Answer from the drawing. Dimensions are ordinates in mm from the lowest x, y and z of the part. Round coordinates to 2 decimals unless told otherwise and drop trailing zeros. Write each loop counter-clockwise with the first axis right and the second up, starting at its lowest first coordinate (ties: lowest second). Pieces come first, ordered by that corner, then holes.
1. Flat-ended cylindrical pins translate along their axes: pin 1 Ø3.5 at (x, z) = (4, 13) entering from +Y; pin 2 Ø1.8 at (x, z) = (4, 23) entering from -Y. Find the tip coordinate at first contact, or state that the pin passes through.
2. Straight lines are drawn through the part: probe 1 along X at (y, z) = (3.5, 13); probe 2 along Z at (x, y) = (4, 3); probe 3 along Z at (x, y) = (3.25, 5.5). For each, find the intervals that lie inside material, in ascending order.
3. Find section C-C (y = 2.5). Write down the section's boundary in (x, z).
4. Find section A-A (z = 13). Write down the section's boundary in (x, y).
5. Find section B-B (x = 4). Write down the section's boundary in (y, z), and give its area (3 significant figures).
6. Determine the mould class of the marked faces 1, 2, 3 and 4 for opening direction X: pulls with the +X half, pulls with the -X half, needs draft (parallel to the pull), parting line crosses it, or undercut.
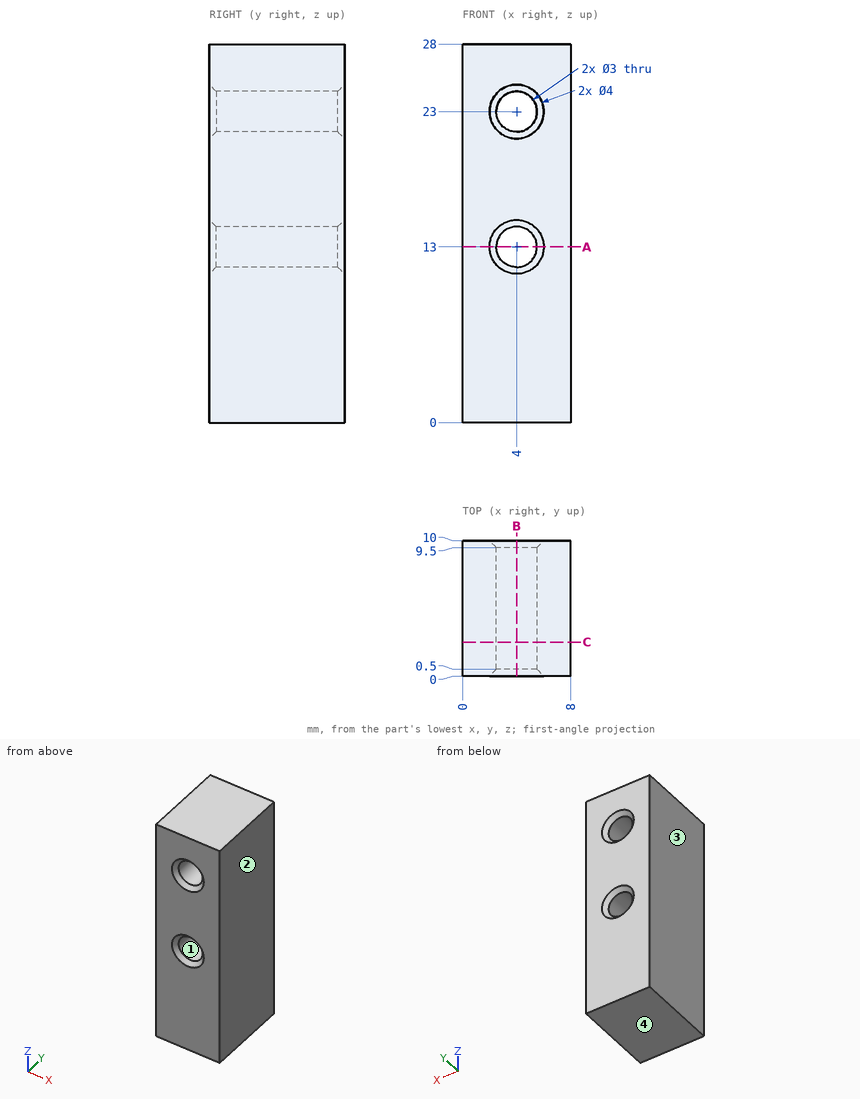
Worked answers:
1. pin 1: stops at y = 9.75
1. pin 2: passes through
2. probe 1: x = 0 to 2.5, 5.5 to 8
2. probe 2: z = 0 to 11.5, 14.5 to 21.5, 24.5 to 28
2. probe 3: z = 0 to 11.7, 14.3 to 21.7, 24.3 to 28
3. outline: (0, 0) - (8, 0) - (8, 28) - (0, 28) - close; hole circle Ø3 at (4, 13); hole circle Ø3 at (4, 23)
4. outline: (0, 0) - (2, 0) - (2.5, 0.5) - (2.5, 9.5) - (2, 10) - (0, 10) - close; (5.5, 0.5) - (6, 0) - (8, 0) - (8, 10) - (6, 10) - (5.5, 9.5) - close
5. outline: (0, 0) - (10, 0) - (10, 11) - (9.5, 11.5) - (0.5, 11.5) - (0, 11) - close; (0, 15) - (0.5, 14.5) - (9.5, 14.5) - (10, 15) - (10, 21) - (9.5, 21.5) - (0.5, 21.5) - (0, 21) - close; (0, 25) - (0.5, 24.5) - (9.5, 24.5) - (10, 25) - (10, 28) - (0, 28) - close
5. area: 219 mm2
6. face 1: undercut
6. face 2: pulls with the +X half
6. face 3: pulls with the -X half
6. face 4: needs draft
